Work out the finished part from the listing and answer in its coordinate system (mm). A direction names the side the tool comes from. Coordinates: 2 decimals unless noted, no trailing zeros. Write each loop counter-clockwise with the first axis right and the second up, starting at its lowest first coordinate (ties: lowest second). Pieces come first, ordered by that corner, then holes. Notation, with made-up numbers: (-36.75, -25.5) - (-29.75, -25.5) arc R24 ccw to (-29.75, 4.5) - close; hole circle Ø10 at (-31.5, 53.25). An arc over 180 degrees is marked (long way). Use a Markdown table: item, result. Add a question column.
(1) The part is cut by section D-D, the plane y = 2.25. Give the vertices of the cut face in (x, z), then the cut area to 3 significant figures.
(2) The part is cut by section C-C, the plane y = 0.5. Give the vertices of the cut face in (x, z).
(3) The part is cut by section B-B, the plane z = 0. Give the vertices of the cut face in (x, y), then the cut area to 3 significant figures.
(4) Find the intervals of material crossed by line 1 (Z direction, x = 0, y = 5); line 2 (X direction, y = 3.25, z = -5), in increasing order. Write a range as from..to.
(5) Given pin 1 Ø1.5 at (x, y) = (-8.5, 3) entering from -Z; pin 2 Ø4 at (y, z) = (5, 4) entering from -X; pin 3 Ø12.5 at (x, z) = (-3, -2) entering from +Y; pin 4 Ø3 at (y, z) = (5.5, 3.5) entering from +X, each flat-ended and moving along its own axis, determine where each tip first touches the part or whether it passes through.
(6) The part is cut by section A-A, the plane x = 0. Give the vertices of the cut face in (y, z), then the cut area to 3 significant figures.
(7) For a pull along X with two mould halves and no side action, classify faces 3 (the face through (-2.7, 6.2, 12)), 4 (the face through (5.97, 3.45, -9.36)), 5 (the face through (-3, 0, -11)) as released by +X, released by -X, zero draft, split by the parting line, or undercut.
(8) A tool of negligible diameter and unlimited length cuts with its end or side. For faces 1 (the face through (-6.42, 3.53, -10.08)), 2 (the face through (-3, 7, -11)), from which of +Z, -Z, +X, -X, +Y, -Y can it reach the whole face along a straight path? Write none if from no direction.
from build123d import *

# Parameters (mm, degrees)
SKETCH1_R           = 12.3
SKETCH1_R_2         = 11.1
BOSS_EXTRUDE1_DEPTH = 7
SKETCH2_W           = 0.35
SKETCH2_H           = 4


with BuildPart() as part:
    # Sketch1 → Boss-Extrude1 (new body)
    with BuildSketch(Plane(origin=(0, 0, 0), x_dir=(1, 0, 0), z_dir=(0, 1, 0))):
        Circle(SKETCH1_R)
        Circle(SKETCH1_R_2, mode=Mode.SUBTRACT)
    extrude(amount=BOSS_EXTRUDE1_DEPTH)

    # Sketch2 → Cut-Revolve1 (revolve, cut)
    with BuildSketch(Plane.XY):
        with Locations((-12.125, 3.5)):
            Rectangle(SKETCH2_W, SKETCH2_H)
    revolve(axis=Axis((0, 7, 0), (0, -1, 0)), mode=Mode.SUBTRACT)


solid = part.part
Model answer:
| question | item | result |
|---|---|---|
| 1 | outline | circle Ø23.9 at (0, 0); hole circle Ø22.2 at (0, 0) |
| 1 | area | 61.6 mm^2 |
| 2 | outline | circle Ø24.6 at (0, 0); hole circle Ø22.2 at (0, 0) |
| 3 | outline | (-12.3, 0) - (-11.1, 0) - (-11.1, 7) - (-12.3, 7) - (-12.3, 5.5) - (-11.95, 5.5) - (-11.95, 1.5) - (-12.3, 1.5) - close; (11.1, 0) - (12.3, 0) - (12.3, 1.5) - (11.95, 1.5) - (11.95, 5.5) - (12.3, 5.5) - (12.3, 7) - (11.1, 7) - close |
| 3 | area | 14.0 mm^2 |
| 4 | line 1 | -11.95..-11.1, 11.1..11.95 |
| 4 | line 2 | -10.85..-9.91, 9.91..10.85 |
| 5 | pin 1 | z = -9.1 |
| 5 | pin 2 | x = -12.13 |
| 5 | pin 3 | through |
| 5 | pin 4 | x = 12.14 |
| 6 | outline | (0, -12.3) - (1.5, -12.3) - (1.5, -11.95) - (5.5, -11.95) - (5.5, -12.3) - (7, -12.3) - (7, -11.1) - (0, -11.1) - close; (0, 11.1) - (7, 11.1) - (7, 12.3) - (5.5, 12.3) - (5.5, 11.95) - (1.5, 11.95) - (1.5, 12.3) - (0, 12.3) - close |
| 6 | area | 14.0 mm^2 |
| 7 | face 3 | split by the parting line |
| 7 | face 4 | undercut |
| 7 | face 5 | zero draft |
| 8 | face 1 | none |
| 8 | face 2 | +Z, -Z, +X, -X, +Y |
